from build123d import *

# Parameters (mm, degrees)
BOSS_EXTRUDE1_DEPTH = 3.000000096
SKETCH2_R           = 3.175
CUT_EXTRUDE1_DEPTH  = 4.000000096
SKETCH3_W           = 2.54
SKETCH3_H           = 0.635
SKETCH3_W_2         = 12.7
SKETCH3_H_2         = 2.201822509
SKETCH3_W_3         = 0.635
SKETCH3_H_3         = 2.54
CUT_EXTRUDE2_DEPTH  = 4.000000096


with BuildPart() as part:
    # Sketch1 → Boss-Extrude1 (new body)
    with BuildSketch(Plane.XY):
        with BuildLine():
            Line((8.696654013, 17.676910134), (34.405475059, 43.38573118))
            ThreePointArc((34.405475059, 43.38573118), (21.189947017, 51.157057474), (6.35, 55.006689448))
            Line((6.35, 55.006689448), (6.35, 18.648926052))
            Line((6.35, 18.648926052), (4.88230096, 15.105587123))
            ThreePointArc((4.88230096, 15.105587123), (-6.075099489, 14.666587579), (-14.133571205, 7.228954972))
            Line((-14.133571205, 7.228954972), (-17.676910134, 8.696654013))
            Line((-17.676910134, 8.696654013), (-76.191723231, 67.21146711))
            ThreePointArc((-76.191723231, 67.21146711), (-38.880636728, 93.866160503), (6.35, 101.401368334))
            Line((6.35, 101.401368334), (6.35, 67.775177491))
            ThreePointArc((6.35, 67.775177491), (26.050026608, 62.890327537), (43.43415954, 52.414415661))
            Line((43.43415954, 52.414415661), (67.21146711, 76.191723231))
            ThreePointArc((67.21146711, 76.191723231), (93.866160503, 38.880636728), (101.401368334, -6.35))
            Line((101.401368334, -6.35), (18.648926052, -6.35))
            Line((18.648926052, -6.35), (15.105587123, -4.88230096))
            ThreePointArc((15.105587123, -4.88230096), (14.666587579, 6.075099489), (7.228954972, 14.133571205))
            Line((7.228954972, 14.133571205), (8.696654013, 17.676910134))
        make_face()
        with BuildLine():
            Line((88.672924278, 6.35), (27.86051193, 6.35))
            ThreePointArc((27.86051193, 6.35), (26.399857642, 10.93517908), (24.190484974, 15.210228852))
            Line((24.190484974, 15.210228852), (67.191354125, 58.211098004))
            ThreePointArc((67.191354125, 58.211098004), (82.13289044, 34.020557137), (88.672924278, 6.35))
        make_face(mode=Mode.SUBTRACT)
        with BuildLine():
            Line((-58.211098004, 67.191354125), (-15.210228852, 24.190484974))
            ThreePointArc((-15.210228852, 24.190484974), (-10.93517908, 26.399857642), (-6.35, 27.86051193))
            Line((-6.35, 27.86051193), (-6.35, 88.672924278))
            ThreePointArc((-6.35, 88.672924278), (-34.020557137, 82.13289044), (-58.211098004, 67.191354125))
        make_face(mode=Mode.SUBTRACT)
    extrude(amount=BOSS_EXTRUDE1_DEPTH)

    # Sketch2 → Cut-Extrude1 (cut, through all)
    with BuildSketch(Plane.XY.offset(3.000000096)):
        with Locations((22.225, 0)):
            Circle(SKETCH2_R)
        with Locations((36.195, 0)):
            Circle(SKETCH2_R)
        with Locations((61.722, 0)):
            Circle(SKETCH2_R)
        with Locations((75.692, 0)):
            Circle(SKETCH2_R)
        with Locations((95.25, 0)):
            Circle(SKETCH2_R)
        with Locations((15.715448212, 15.715448212)):
            Circle(SKETCH2_R)
        with Locations((25.593729945, 25.593729945)):
            Circle(SKETCH2_R)
        with Locations((43.644044748, 43.644044748)):
            Circle(SKETCH2_R)
        with Locations((53.522326482, 53.522326482)):
            Circle(SKETCH2_R)
        with Locations((92.004434954, 24.652514046)):
            Circle(SKETCH2_R)
        with Locations((82.48891971, 47.625)):
            Circle(SKETCH2_R)
        with Locations((67.351920908, 67.351920908)):
            Circle(SKETCH2_R)
        with Locations((0, 95.25)):
            Circle(SKETCH2_R)
        with Locations((0, 75.692)):
            Circle(SKETCH2_R)
        with Locations((-53.522326482, 53.522326482)):
            Circle(SKETCH2_R)
        with Locations((-43.644044748, 43.644044748)):
            Circle(SKETCH2_R)
        with Locations((0, 61.722)):
            Circle(SKETCH2_R)
        with Locations((0, 36.195)):
            Circle(SKETCH2_R)
        with Locations((-25.593729945, 25.593729945)):
            Circle(SKETCH2_R)
        with Locations((-15.715448212, 15.715448212)):
            Circle(SKETCH2_R)
        with Locations((0, 22.225)):
            Circle(SKETCH2_R)
        with Locations((-24.652514046, 92.004434954)):
            Circle(SKETCH2_R)
        with Locations((-47.625, 82.48891971)):
            Circle(SKETCH2_R)
        with Locations((-67.351920908, 67.351920908)):
            Circle(SKETCH2_R)
    extrude(amount=-CUT_EXTRUDE1_DEPTH, mode=Mode.SUBTRACT)

    # Sketch3 → Cut-Extrude2 (cut, through all)
    with BuildSketch(Plane.XY.offset(3.000000096)):
        Polygon((15.266435406, 24.246691527), (17.06248663, 26.042742751), (17.511499436, 25.593729945), (15.715448212, 23.797678721), align=None)
        Polygon((55.048970022, 64.029226143), (56.845021246, 65.825277367), (57.294034052, 65.376264561), (55.497982828, 63.580213337), align=None)
        Polygon((29.230733674, 38.210989795), (31.026784898, 40.007041019), (40.007041019, 31.026784898), (38.210989795, 29.230733674), align=None)
        with Locations((29.21, -6.0325)):
            Rectangle(SKETCH3_W, SKETCH3_H)
        with Locations((68.707, -6.0325)):
            Rectangle(SKETCH3_W, SKETCH3_H)
        Polygon((43.43415954, 52.414415661), (44.991083167, 53.971339288), (45.440095973, 53.522326482), (43.883172346, 51.965402855), align=None)
        with Locations((48.9585, -6.0325)):
            Rectangle(SKETCH3_W, SKETCH3_H)
        with Locations((85.471, -6.0325)):
            Rectangle(SKETCH3_W, SKETCH3_H)
        Polygon((99.935462164, 14.437711971), (100.266998693, 11.919442024), (101.526133667, 12.085210288), (101.194597138, 14.603480236), align=None)
        Polygon((93.765504959, 37.464305742), (94.938831965, 37.950313702), (93.966816047, 40.296967714), (92.793489041, 39.810959755), align=None)
        Polygon((79.327792988, 62.471156422), (80.874047017, 60.456038938), (81.88160576, 61.229165953), (80.33535173, 63.244283437), align=None)
        Polygon((13.593916116, 7.005422516), (14.565932035, 4.658768503), (15.739259041, 5.144776462), (14.767243123, 7.491430475), align=None)
        with Locations((0, 68.876088745)):
            Rectangle(SKETCH3_W_2, SKETCH3_H_2)
        Polygon((-40.007041019, 31.026784898), (-38.210989795, 29.230733674), (-37.761976989, 29.67974648), (-39.558028213, 31.475797704), align=None)
        Polygon((-26.042742751, 17.06248663), (-25.593729945, 17.511499436), (-23.797678721, 15.715448212), (-24.246691527, 15.266435406), align=None)
        Polygon((-65.825277367, 56.845021246), (-64.029226143, 55.048970022), (-63.580213337, 55.497982828), (-65.376264561, 57.294034052), align=None)
        Polygon((-63.244283437, 80.33535173), (-61.229165953, 81.88160576), (-60.456038938, 80.874047017), (-62.471156422, 79.327792988), align=None)
        Polygon((-37.950313702, 94.938831965), (-40.296967714, 93.966816047), (-39.810959755, 92.793489041), (-37.464305742, 93.765504959), align=None)
        Polygon((-14.437711971, 99.935462165), (-14.603480236, 101.194597138), (-12.085210288, 101.526133667), (-11.919442024, 100.266998693), align=None)
        with Locations((6.0325, 85.471)):
            Rectangle(SKETCH3_W_3, SKETCH3_H_3)
        with Locations((6.0325, 48.9585)):
            Rectangle(SKETCH3_W_3, SKETCH3_H_3)
        with Locations((6.0325, 29.21)):
            Rectangle(SKETCH3_W_3, SKETCH3_H_3)
        Polygon((-7.491430475, 14.767243123), (-5.144776462, 15.739259041), (-4.658768503, 14.565932035), (-7.005422516, 13.593916116), align=None)
        Polygon((-53.971339288, 44.991083167), (-52.175288063, 43.195031942), (-51.726275257, 43.644044748), (-53.522326482, 45.440095973), align=None)
    extrude(amount=-CUT_EXTRUDE2_DEPTH, mode=Mode.SUBTRACT)


solid = part.part
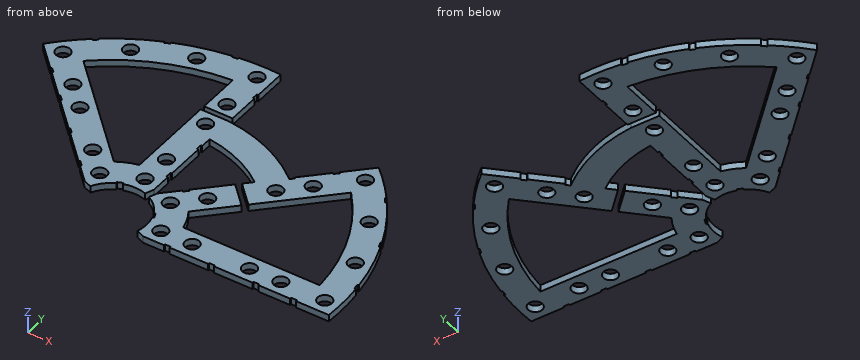
Read the model definition and answer for the solid it produces. Units are mm, in the model's axes. Give positions to 0.01 mm unless a question says otherwise; leave off trailing zeros. Loops run counter-clockwise (first coordinate to the right, second up) from the corner with the lowest first, then second, coordinate; pieces in that order, holes last. Notation, with made-up numbers: M 7.25,42 L 59.25,42 A17 ccw 59.25,47 Z; hole C 80,38.25 d3. An arc over 180 degrees is marked long. Write each question's results on one line, items separated by ' | '.
1. Straight lines are drawn through the part: line 1 (Y direction, x = -17, z = 2.35); line 2 (X direction, y = 47, z = 1.5); line 3 (X direction, y = 40, z = 2.25). For each, find the intervals that lie inside material, in ascending order. Write a range as [from, to].
Values:
line 1: y = [8.42, 12.81], [18.62, 25.98], [87.26, 100.17] | line 2: x = [-55.98, -38.02], [-6.35, 6.35], [29.28, 55.98], [75.46, 79.38], [85.6, 90.08] | line 3: x = [-48.98, -31.02], [-6.35, 6.35], [31.03, 48.98], [79.39, 93.25]
2. Section A-A on x = 0 is taken. Give the vertices of the cut face in (y, z) (3 decimals).
Values:
outline: M 15.875,0 L 19.05,0 L 19.05,3 L 15.875,3 Z; M 25.4,0 L 33.02,0 L 33.02,3 L 25.4,3 Z; M 39.37,0 L 58.547,0 L 58.547,3 L 39.37,3 Z; M 64.897,0 L 67.775,0 L 67.775,3 L 64.897,3 Z; M 69.977,0 L 72.517,0 L 72.517,3 L 69.977,3 Z; M 78.867,0 L 92.075,0 L 92.075,3 L 78.867,3 Z; M 98.425,0 L 101.6,0 L 101.6,3 L 98.425,3 Z
3. Section B-B on y = 0 is taken. Give the vertices of the cut face in (x, z) (3 decimals).
Values:
outline: M 15.875,0 L 19.05,0 L 19.05,3 L 15.875,3 Z; M 25.4,0 L 33.02,0 L 33.02,3 L 25.4,3 Z; M 39.37,0 L 58.547,0 L 58.547,3 L 39.37,3 Z; M 64.897,0 L 72.517,0 L 72.517,3 L 64.897,3 Z; M 78.867,0 L 92.075,0 L 92.075,3 L 78.867,3 Z; M 98.425,0 L 101.6,0 L 101.6,3 L 98.425,3 Z
4. Section C-C on z = 1.4 is taken. State how many separate pieces and enclosed holes the cut face has, plus the area to 3 significant figures.
Values:
separate pieces: 1 | enclosed holes: 24 | area: 5,650 mm^2
5. Given pin 1 (0.7 mm diameter, centred on y = -6, z = 2, fed in from -X); pin 2 (0.8 mm diameter, centred on x = 68.5, z = 2, fed in from -Y) (3 decimals); pin 3 (0.9 mm diameter, centred on x = 2.5, z = 1, fed in from -Y), each flat-ended and moving along its own axis, determine where each tip first touches the part or whether it passes through.
Values:
pin 1: stops at x = 16.96 | pin 2: stops at y = -5.715 | pin 3: stops at y = 15.6
